Autodesk Inventor part; units mm, degrees
ref_plane "YZ Plane" through (0, 0, 0) normal (1, 0, 0) x (0, 1, 0)
ref_plane "XZ Plane" through (0, 0, 0) normal (0, 1, 0) x (-1, 0, 0)
ref_plane "XY Plane" through (0, 0, 0) normal (0, 0, 1) x (1, 0, 0)
sketch "Sketch1" plane through (0, 0, 0) normal (0, 0, 1) x (1, 0, 0)
  line L0 (2.8868, 0) -> (1.4434, -2.5)
  line L1 (1.4434, -2.5) -> (-1.4434, -2.5)
  line L2 (-1.4434, -2.5) -> (-2.8868, 0)
  line L3 (-2.8868, 0) -> (-1.4434, 2.5)
  line L4 (-1.4434, 2.5) -> (1.4434, 2.5)
  line L5 (1.4434, 2.5) -> (2.8868, 0)
  point P0 (0, 0)
  point P1 (0, 0)
  dimension "d0" = 5
extrude "Extrusion1" add sketch "Sketch1" along normal blind 10
sketch "Sketch2" plane through (0, 0, 10) normal (0, 0, 1) x (1, 0, 0)
  circle A0 centre (0, 0) radius 1.5
  dimension "d3" = 3
extrude "Extrusion2" add sketch "Sketch2" along normal blind 6
sketch "Sketch3" plane through (0, 0, 0) normal (0, 0, -1) x (-1, 0, 0)
  circle A0 centre (0, 0) radius 1.5
  dimension "d6" = 3
extrude "Extrusion3" cut sketch "Sketch3" against normal blind 4
properties part number "Spacer7mm_m3"
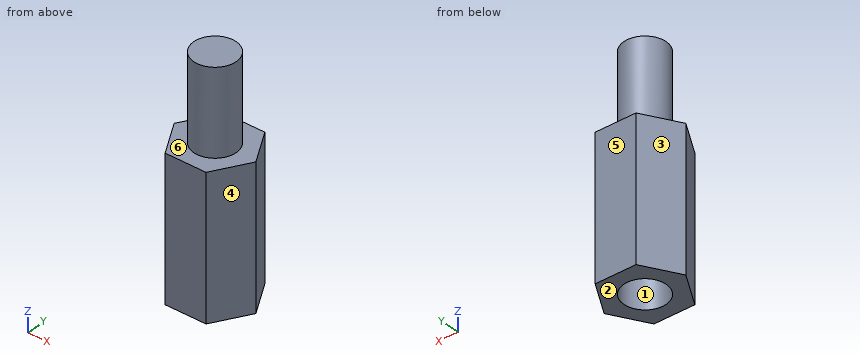
Part model, mm, in its own coordinate system. Face numbers are marked on the shaded views. A direction names the side the tool comes from. Coordinates: 2 decimals unless noted, no trailing zeros. Order: outer loops, then holes, each group sorted by start corner. A loop starts at its lowest first (then second) coordinate and runs counter-clockwise, first axis right, second up. Notation, with made-up numbers: M 23,13.25 L 36,13.25 A28 cw 36,32.25 Z; hole C 78,-20.5 d4. An arc over 180 degrees is marked long. One line per question, with ' | ' between items.
Q1. Slice it at C-C (y = 0.8). Give the cut face in (x, z), and give its area (3 significant figures).
A:
outline: M -2.42,0 L -1.27,0 L -1.27,4 L 1.27,4 L 1.27,0 L 2.42,0 L 2.42,10 L 1.27,10 L 1.27,16 L -1.27,16 L -1.27,10 L -2.42,10 Z | area: 53.6 mm^2
Q2. Drill centre lines: line 1 (Y direction, x = 0, z = 1.55); line 2 (Z direction, x = 2.05, y = -0.25); line 3 (Z direction, x = -1.15, y = -0.25). Where is each one in solid material? Low to high.
A:
line 1: y = -2.5 to -1.5, 1.5 to 2.5 | line 2: z = 0 to 10 | line 3: z = 4 to 16
Q3. Two-plate mould, pull along X, no slides. Class the marked faces 1, 2, 3 and 4: +X half, -X half, draft (parallel to the pull), parting line (faces both ways), or undercut.
A:
face 1: undercut | face 2: draft | face 3: -X half | face 4: +X half
Q4. Slice it at B-B (z = 2.5). Give the cut face in (x, y), and give its area (3 significant figures).
A:
outline: M -2.89,0 L -1.44,-2.5 L 1.44,-2.5 L 2.89,0 L 1.44,2.5 L -1.44,2.5 Z; hole C 0,0 d3 | area: 14.6 mm^2
Q5. 3-axis set-ups, long thin cutter, end or side, ignore diameter. For the marked faces 5 and 6: which of +Z, -Z, +X, -X, +Y, -Y reach the whole face in a straight line?
A:
face 5: +Z, -Z, +X, -X, +Y | face 6: +Z
Q6. Pin check, flat tips, straight feed: P1, Ø1.5, axis at x = -0.5, y = -0.5, coming from the -Z side; P2, Ø3, axis at y = 1, z = 7, coming from the -X side. Stop position of each tip, or through.
A:
P1: stops at z = 4 | P2: stops at x = -2.89
Q7. Slice it at D-D (z = 8.75). Give the cut face in (x, y), and give its area (3 significant figures).
A:
outline: M -2.89,0 L -1.44,-2.5 L 1.44,-2.5 L 2.89,0 L 1.44,2.5 L -1.44,2.5 Z | area: 21.7 mm^2
Q8. Slice it at A-A (x = 0). Give the cut face in (y, z), and give its area (3 significant figures).
A:
outline: M -2.5,0 L -1.5,0 L -1.5,4 L 1.5,4 L 1.5,0 L 2.5,0 L 2.5,10 L 1.5,10 L 1.5,16 L -1.5,16 L -1.5,10 L -2.5,10 Z | area: 56.0 mm^2
